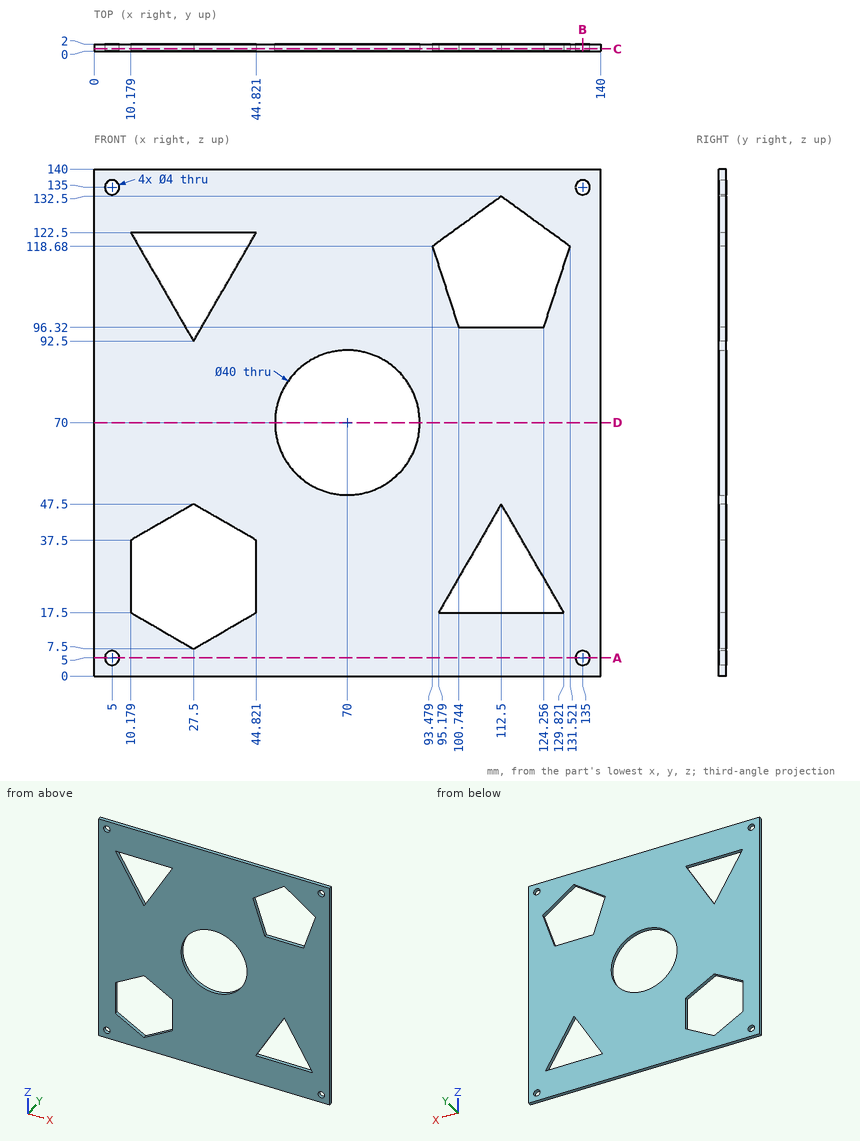
Geometry check sheet. Reference: drawing and pictorial views, mm from the part's lowest x, y, z. Give positions to 0.01 mm unless a question says otherwise; leave off trailing zeros. Loops run counter-clockwise (first coordinate to the right, second up) from the corner with the lowest first, then second, coordinate; pieces in that order, holes last. Notation, with made-up numbers: (-35, -28.5) - (-16, -28.5) arc R18 cw to (-16, 3.5) - close; hole circle Ø8 at (-23, -34). An arc over 180 degrees is marked (long way). One line per question, with ' | ' between items. Start each with the question number.
1. Material ranges on line 1 along Z through (x, y) = (135, 0.95); line 2 along X through (y, z) = (1, 113) (1 decimal), recorded low to high. Write a range as [from, to].
2. Cross-section at B-B, the plane x = 135. Enter the section's corners in (y, z), plus the area to 3 significant figures.
3. Cross-section at D-D, the plane z = 70. Enter the section's corners in (x, y), plus the area to 3 significant figures.
4. Gauge pin test, flat end, axial feed: pin 1 Ø10 at (x, z) = (77, 58) entering from +Y. Record the tip position at first contact, or that the pin passes through.
5. Cross-section at C-C, the plane y = 0.65. Give the number of separate pieces and of enclosed holes in the cut face, plus the area to 3 significant figures.
6. Cross-section at A-A, the plane z = 5. Enter the section's corners in (x, y), plus the area to 3 significant figures.
Check result:
1) line 1: z = [0, 3], [7, 133], [137, 140] | line 2: x = [0, 15.7], [39.3, 95.3], [129.7, 140]
2) outline: (0, 0) - (2, 0) - (2, 3) - (0, 3) - close; (0, 7) - (2, 7) - (2, 133) - (0, 133) - close; (0, 137) - (2, 137) - (2, 140) - (0, 140) - close | area: 264 mm2
3) outline: (0, 0) - (50, 0) - (50, 2) - (0, 2) - close; (90, 0) - (140, 0) - (140, 2) - (90, 2) - close | area: 200 mm2
4) pin 1: passes through
5) separate pieces: 1 | enclosed holes: 9 | area: 15,300 mm2
6) outline: (0, 0) - (3, 0) - (3, 2) - (0, 2) - close; (7, 0) - (133, 0) - (133, 2) - (7, 2) - close; (137, 0) - (140, 0) - (140, 2) - (137, 2) - close | area: 264 mm2
